from build123d import *

# Parameters (mm, degrees)
F0_R     = 16
F0_R_2   = 10
F1_DEPTH = 42
F2_R     = 0.25
F4_START = -5.75
F3_R     = 16
F3_R_2   = 15.25
F4_DEPTH = 1.6
F5_START = -34.65
F5_DEPTH = 1.6


with BuildPart() as f1:
    # F0 (on Top) → F1 (new body)
    with BuildSketch(Plane.XY):
        Circle(F0_R)
        Circle(F0_R_2, mode=Mode.SUBTRACT)
    extrude(amount=F1_DEPTH)

    # F2
    f2_edges = [f1.edges().sort_by_distance(p)[0] for p in [
        (-16, 0, 42),
        (-10, 0, 42),
        (-16, 0, 0),
        (-10, 0, 0),
    ]]
    fillet(f2_edges, radius=F2_R)

    # F3 (on face) → F4 (cut)
    with BuildSketch(Plane.XY.offset(42).offset(F4_START)):
        Circle(F3_R)
        Circle(F3_R_2, mode=Mode.SUBTRACT)
    extrude(amount=-F4_DEPTH, mode=Mode.SUBTRACT)

    # F3 (on face) → F5 (cut)
    with BuildSketch(Plane.XY.offset(42).offset(F5_START)):
        Circle(F3_R)
        Circle(F3_R_2, mode=Mode.SUBTRACT)
    extrude(amount=-F5_DEPTH, mode=Mode.SUBTRACT)


solid = f1.part
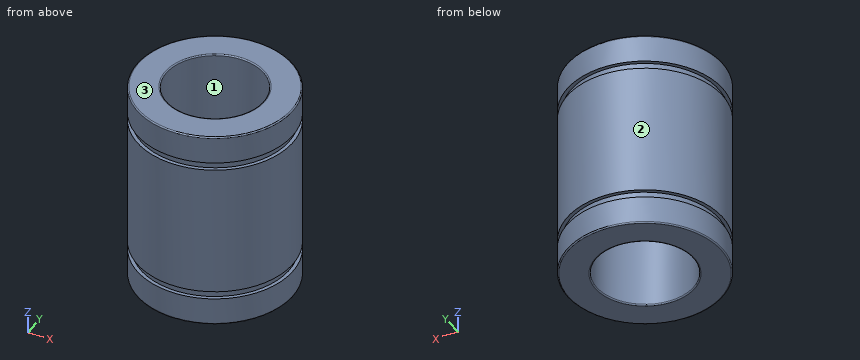
Can you work these out from the model? Positions are in its coordinate system, mm. Face numbers are marked on the shaded views. Give positions to 0.01 mm unless a question says otherwise; leave off trailing zeros. Loops run counter-clockwise (first coordinate to the right, second up) from the corner with the lowest first, then second, coordinate; pieces in that order, holes last. Notation, with made-up numbers: M 58.25,22 L 103.25,22 A30 ccw 103.25,52 Z; hole C 68,61.25 d7. An arc over 180 degrees is marked long. One line per item, written item: value. Start each with the question number.
1) If I drill on line 1 (Z direction, x = 4.5, y = 15); line 2 (Y direction, x = 0, z = 28); line 3 (X direction, y = 12.5, z = 25.5), over which ranges is the centre line in solid material (lowest first)? Write a range as [from, to].
2) Thinking about a two-plate mould opening in X: for the marked faces 1, 2 and 3, which applies, +X half, -X half, draft (parallel to the pull), parting line (faces both ways), or undercut?
3) If we section it at C-C, the plane z = 28.5: Write out the boundary of the cut face in (x, y).
4) I'm going to push flat-ended pins straight in: pin 1 (1 mm diameter, centred on x = -3.5, z = 5, fed in from +Y); pin 2 (4 mm diameter, centred on y = -6, z = 34, fed in from -X); pin 3 (3 mm diameter, centred on x = 1.5, z = 11, fed in from -Y); pin 4 (16 mm diameter, centred on x = 0, y = 0, fed in from +Z). Where does each tip first touch, or does it pass through?
Completed:
1. line 1: z = [0, 5.75], [7.35, 34.65], [36.25, 42]
1. line 2: y = [-16, -10], [10, 16]
1. line 3: x = [-9.99, 9.99]
2. face 1: undercut
2. face 2: parting line
2. face 3: draft
3. outline: C 0,0 d32; hole C 0,0 d20
4. pin 1: stops at y = 15.72
4. pin 2: stops at x = -15.49
4. pin 3: stops at y = -16
4. pin 4: passes through
